```python
from build123d import *

# Parameters (mm, degrees)
F1_DEPTH = 75
F2_DEPTH = 4
F3_DEPTH = 200
F4_DEPTH = 10


with BuildPart() as f1:
    # F0 (on Right) → F1 (new body, symmetric)
    with BuildSketch(Plane.YZ):
        with BuildLine():
            Line((-92.3375381151, 150), (-58.3594357527, 150))
            ThreePointArc((-58.3594357527, 150), (-62.8590677445, 219.5182916975), (-46.5160623858, 287.2379029225))
            add(Edge.make_bspline(
                [(-92.3375381151, 150), (-83.8972050592, 197.0286155209), (-65.4330781641, 242.1901230497), (-46.5160623858, 287.2379029225)],
                knots=[0.5005259003, 0.5005259003, 0.5005259003, 0.5005259003, 0.9842554423, 0.9842554423, 0.9842554423, 0.9842554423], degree=3))
        make_face()
        with BuildLine():
            Line((-97.0230517394, 0), (50.0025975795, 0))
            ThreePointArc((50.0025975795, 0), (-19.782437401, 63.7274456487), (-58.3594357527, 150))
            Line((-58.3594357527, 150), (-92.3375381151, 150))
            add(Edge.make_bspline(
                [(-97.0230517394, 0), (-99.0723612734, 50.6778343669), (-101.0709416697, 101.3384276147), (-92.3375381151, 150)],
                knots=[0, 0, 0, 0, 0.5005259003, 0.5005259003, 0.5005259003, 0.5005259003], degree=3))
        make_face()
        with BuildLine():
            Line((-58.3594357527, 150), (-35.7824824753, 150))
            ThreePointArc((-35.7824824753, 150), (9.701095737, 337.2321487603), (188.6912309552, 408.5565128374))
            Line((188.6912309552, 408.5565128374), (190.8316842979, 408.5565128374))
            Line((190.8316842979, 408.5565128374), (190.8316842979, 430.4521389342))
            ThreePointArc((190.8316842979, 430.4521389342), (50.4625001931, 399.417827924), (-44.6678048686, 291.636283284))
            add(Edge.make_bspline(
                [(-46.5160623858, 287.2379029225), (-45.9003463268, 288.7041300386), (-45.284150482, 290.1702366729), (-44.6678048686, 291.636283284)],
                knots=[0.9842554423, 0.9842554423, 0.9842554423, 0.9842554423, 1, 1, 1, 1], degree=3))
            ThreePointArc((-46.5160623858, 287.2379029225), (-62.8590677445, 219.5182916975), (-58.3594357527, 150))
        make_face()
        with BuildLine():
            Line((50.0025975795, 0), (102.9769482606, 0))
            ThreePointArc((102.9769482606, 0), (14.1204583697, 56.9827590308), (-35.7824824753, 150))
            Line((-35.7824824753, 150), (-58.3594357527, 150))
            ThreePointArc((-58.3594357527, 150), (-19.782437401, 63.7274456487), (50.0025975795, 0))
        make_face()
    extrude(amount=F1_DEPTH, both=True)

    # F2 (add): a face of the model
    f2_faces = [f1.faces().sort_by_distance(p)[0] for p in [
        (0, 2.9769482606, 0),
    ]]
    extrude(f2_faces, amount=F2_DEPTH)

    # F3 (add): a face of the model
    f3_faces = [f1.faces().sort_by_distance(p)[0] for p in [
        (0, -97.0230517394, -2),
    ]]
    extrude(f3_faces, amount=F3_DEPTH)

    # F4 (add): a face of the model
    f4_faces = [f1.faces().sort_by_distance(p)[0] for p in [
        (0, -197.0230517394, 0),
    ]]
    extrude(f4_faces, amount=F4_DEPTH)


solid = f1.part
```
The listing builds one solid part. Answer for the finished solid, in the listing's coordinates (mm). Round coordinates to 2 decimals unless told otherwise and drop trailing zeros. Write each loop counter-clockwise with the first axis right and the second up, starting at its lowest first coordinate (ties: lowest second). Pieces come first, ordered by that corner, then holes. Notation, with made-up numbers: (-32, 10) -> (-25, 10) arc R15 cw to (-25, 39) -> close; hole circle Ø2 at (0.5, 63). An arc over 180 degrees is marked (long way). Write item = value, one per line.
1) For a pull along Z with two mould halves and no side action, classify faces 1 (the flat face through (-1, -94, -4)), 2 (the cylindrical face through (1.05, 52.23, 400.45)), 3 (the flat face through (75, -34, 132)), 4 (the cylindrical face through (1.05, -38.083, 238.474)) as released by +Z, released by -Z, zero draft, split by the parting line, or undercut.
Check values:
face_1 = released by -Z
face_2 = released by +Z
face_3 = zero draft
face_4 = undercut
2) Section B-B on z = 303.5 is taken. Write down the section's boundary in (x, y).
Check values:
outline = (-75, -39.14) -> (75, -39.14) -> (75, -14.2) -> (-75, -14.2) -> close
3) Straight lines are drawn through the part: line 1 along Z through (x, y) = (45.5, -224.5); line 2 along Z through (x, y) = (-41.5, 71); line 3 along Z through (x, y) = (-39, 95). For each, find the intervals that lie inside material, in ascending order. Write a range as [from, to].
Check values:
line_1 = [-4, 10]
line_2 = [-4, 13.48], [385.67, 410.18]
line_3 = [-4, 2.79], [396.36, 419.68]
4) Section C-C on y = -142 is taken. Write down the section's boundary in (x, z).
Check values:
outline = (-75, -4) -> (75, -4) -> (75, 10) -> (-75, 10) -> close
5) Section A-A on y = 49 is taken. Write down the section's boundary in (x, z).
Check values:
outline = (-75, -4) -> (75, -4) -> (75, 26.75) -> (-75, 26.75) -> close; (-75, 372.4) -> (75, 372.4) -> (75, 398.55) -> (-75, 398.55) -> close
6) Given pin 1 (6 mm diameter, centred on x = -39.5, z = 340, fed in from -Y); pin 2 (1.5 mm diameter, centred on x = -19.5, z = 338.5, fed in from +Y); pin 3 (1 mm diameter, centred on x = -11, z = 346, fed in from -Y), each flat-ended and moving along its own axis, determine where each tip first touches the part or whether it passes through.
Check values:
pin_1 = -18.63
pin_2 = 11.48
pin_3 = -12.07
